```python
from build123d import *

# Parameters (mm, degrees)
BOSS_EXTRUDE1_DEPTH = 400
SKETCH2_R           = 3.25
CUT_EXTRUDE1_DEPTH  = 300


with BuildPart() as part:
    # Sketch1 → Boss-Extrude1 (new body)
    with BuildSketch(Plane.XY):
        Polygon((28, 0), (30, 0), (30, 20), (0, 20), (0, 0), (2, 0), (2, 18), (28, 18), align=None)
    extrude(amount=BOSS_EXTRUDE1_DEPTH)

    # Sketch2 → Cut-Extrude1 (cut)
    with BuildSketch(Plane(origin=(0, 20, 0), x_dir=(1, 0, 0), z_dir=(0, 1, 0))):
        with Locations(Location((15, -70, 0), (0, 0, 270))):
            Circle(SKETCH2_R)
        with Locations(Location((15, -20, 0), (0, 0, 270))):
            Circle(SKETCH2_R)
    extrude(amount=-CUT_EXTRUDE1_DEPTH, mode=Mode.SUBTRACT)


solid = part.part
```
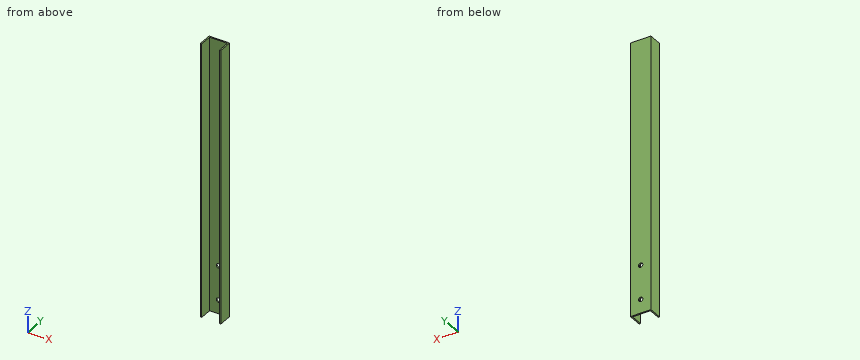
Here's how the part is built. I have some questions about the finished solid (model axes, mm). Give positions to 0.01 mm unless a question says otherwise; leave off trailing zeros. Loops run counter-clockwise (first coordinate to the right, second up) from the corner with the lowest first, then second, coordinate; pieces in that order, holes last. Notation, with made-up numbers: M -29.75,84 L 1.25,84 A20 cw 1.25,99 Z; hole C 10.5,35 d10. An arc over 180 degrees is marked long. Return JSON: item names as keys, results as strings.
Item 1: Imagine slicing it at C-C on z = 338. List the corners of the cut face in (x, y) for me.
A:
{"outline": "M 0,0 L 2,0 L 2,18 L 28,18 L 28,0 L 30,0 L 30,20 L 0,20 Z"}
Item 2: Imagine slicing it at A-A on x = 15. List the corners of the cut face in (y, z) for me.
A:
{"outline": "M 18,0 L 20,0 L 20,16.75 L 18,16.75 Z; M 18,23.25 L 20,23.25 L 20,66.75 L 18,66.75 Z; M 18,73.25 L 20,73.25 L 20,400 L 18,400 Z"}
Item 3: Imagine slicing it at B-B on y = 6.75. List the corners of the cut face in (x, z) for me.
A:
{"outline": "M 0,0 L 2,0 L 2,400 L 0,400 Z; M 28,0 L 30,0 L 30,400 L 28,400 Z"}
Item 4: I'm going to push a flat-ended pin straight in: pin 1 Ø10.5 at (x, z) = (15, 20) entering from -Y. Where does the tip first touch, or does it pass through?
A:
{"pin 1": "stops at y = 18"}
Item 5: Imagine slicing it at D-D on z = 20. List the corners of the cut face in (x, y) for me, then the cut area to 3 significant figures.
A:
{"outline": "M 0,0 L 2,0 L 2,18 L 11.75,18 L 11.75,20 L 0,20 Z; M 18.25,18 L 28,18 L 28,0 L 30,0 L 30,20 L 18.25,20 Z", "area": "119 mm^2"}
Item 6: Please list where these lines run through material, in increasing order: line 1 (X direction, y = 19.55, z = 70); line 2 (X direction, y = 15, z = 240); line 3 (Y direction, x = 24.75, z = 338).
A:
{"line 1": "x = 0 to 11.75, 18.25 to 30", "line 2": "x = 0 to 2, 28 to 30", "line 3": "y = 18 to 20"}
